Geometry: see drawing. Coordinates: mm, zero at the bounding-box minimum. Give positions to 0.01 mm unless a question says otherwise; leave off trailing zeros. Order: outer loops, then holes, each group sorted by start corner. A loop starts at its lowest first (then second) coordinate and runs counter-clockwise, first axis right, second up. Notation, with made-up numbers: (76.25, 13.25) - (129.25, 13.25) arc R33 cw to (129.25, 48.25) - close; hole circle Ø2 at (79.5, 51). An arc over 180 degrees is marked (long way). One line per item, written item: value.
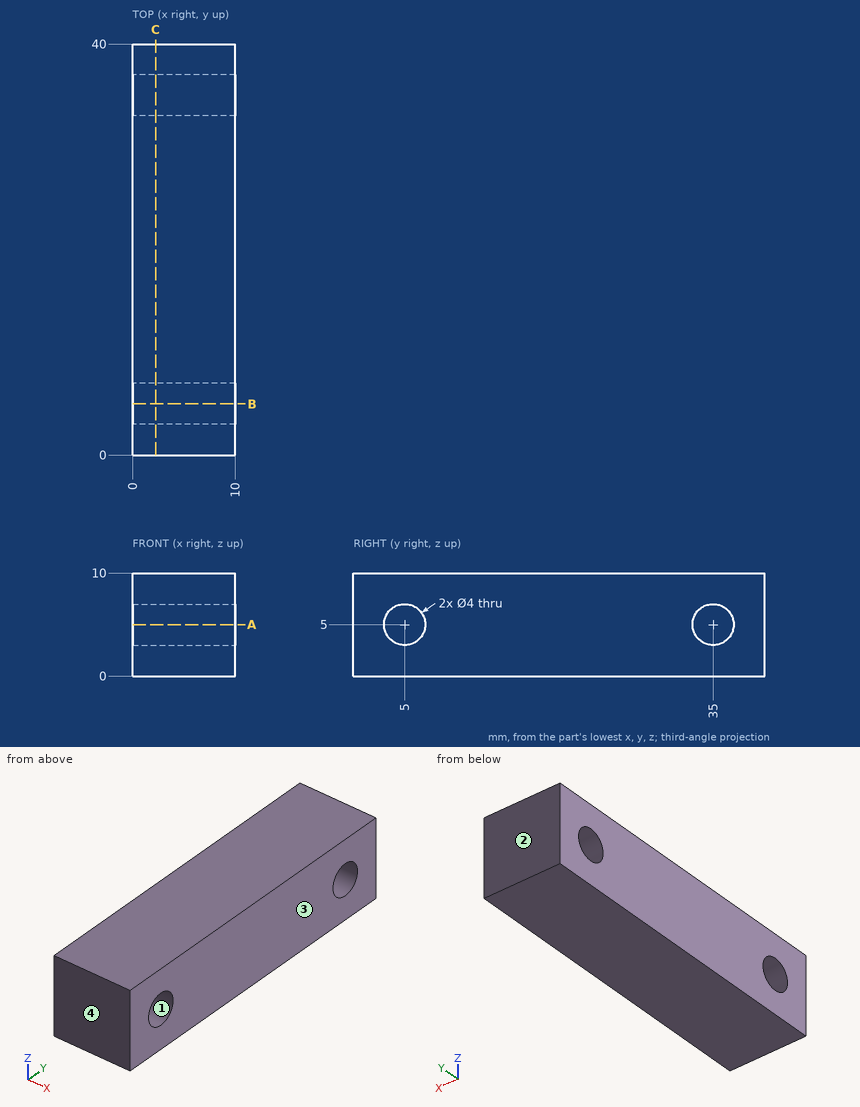
1) Section A-A, the plane z = 5. Return loops of the section in (x, y), then the cut area to 3 significant figures.
Answers below:
outline: (0, 0) - (10, 0) - (10, 3) - (0, 3) - close; (0, 7) - (10, 7) - (10, 33) - (0, 33) - close; (0, 37) - (10, 37) - (10, 40) - (0, 40) - close
area: 320 mm^2
2) Section C-C, the plane x = 2.25. Return loops of the section in (y, z).
Answers below:
outline: (0, 0) - (40, 0) - (40, 10) - (0, 10) - close; hole circle Ø4 at (5, 5); hole circle Ø4 at (35, 5)
3) Mould query, pull axis Y, two halves, no side actions, for the marked faces 1, 2, 3 and 4. Classes: released by +Y, released by -Y, zero draft, split by the parting line, or undercut.
Answers below:
face 1: undercut
face 2: released by +Y
face 3: zero draft
face 4: released by -Y
4) Section B-B, the plane y = 5. Return loops of the section in (x, z).
Answers below:
outline: (0, 0) - (10, 0) - (10, 3) - (0, 3) - close; (0, 7) - (10, 7) - (10, 10) - (0, 10) - close
5) Material intervals for line 1 along Y through (x, z) = (2, 5); line 2 along Y through (x, z) = (2, 5.5); line 3 along Z through (x, y) = (5.75, 5), sorted ascending.
Answers below:
line 1: 0 to 3, 7 to 33, 37 to 40
line 2: 0 to 3.06, 6.94 to 33.06, 36.94 to 40
line 3: 0 to 3, 7 to 10
6) First-contact query: pin 1 (2 mm diameter, centred on x = 3, z = 7.5, fed in from -Y). Flat tip, straight axial feed; report the tip coordinate or a pass-through.
Answers below:
pin 1: y = 0
